Check sheet for the modelled part. Datum: model origin and axes. Units: mm. A direction names the side the tool comes from. Give positions to 0.01 mm unless a question says otherwise; leave off trailing zeros. Write each loop counter-clockwise with the first axis right and the second up, starting at its lowest first coordinate (ties: lowest second). Pieces come first, ordered by that corner, then holes. Notation, with made-up numbers: M 40,13.25 L 66,13.25 A34 ccw 66,49.25 Z; hole C -2.75,4 d3. An arc over 180 degrees is marked long. Use CSV: the item, a comma, the result in double quotes. Start each with the question number.
1. Cross-section at A-A, the plane x = 12. Enter the section's corners in (y, z).
2. Access from +Z, -Z, +X, -X, +Y, -Y to the whole of each face (thin tool, end or side, straight path). Record for faces 4 (the face through (15, 13, -7.62)), 5 (the face through (9.144, 1, -33)), 6 (the face through (19.05, 1, -61)), 7 (the face through (18.84, 21.43, -33.12)), 8 (the face through (8.37, 3.06, -33.12)).
3. Mould release check, pull along X, two halves, no side actions. Record for faces 1 (the face through (31, 3, -7.62)), 2 (the face through (32.84, 1.13, -53.83)), 3 (the face through (7.62, 12, -33)): +X half, -X half, draft (parallel to the pull), parting line (faces both ways), or undercut.
4. Scan lines: line 1 (Z direction, x = 9, y = 17.75); line 2 (Y direction, x = 34.5, z = -22.5); line 3 (X direction, y = 8, z = -40). Record each from-to range of solid material in increasing order.
5. Cross-section at B-B, the plane z = -36. Enter the section's corners in (x, y), and give its area (3 significant figures).
6. Cross-section at D-D, the plane z = -23. Enter the section's corners in (x, y), and give its area (3 significant figures).
7. Cross-section at C-C, the plane x = 5. Enter the section's corners in (y, z).
8. Depth check by flat-ended pin: P1, Ø2.5, axis at x = 29.5, z = -5.5, coming from the +Y side; P2, Ø7, axis at x = 16, y = 14.5, coming from the -Z side; P3, Ø4, axis at x = 4, y = 20, coming from the +Z side; P4, Ø4, axis at y = 9, z = -22.5, coming from the +X side. Enter the tip coordinate at first touch or a pass-through.
from build123d import *

# Parameters (mm, degrees)
BOSS_EXTRUDE2_DEPTH   = 3.81
BOSS_EXTRUDE2_2_DEPTH = 3.81
SKETCH2_3_W           = 39.3827
SKETCH2_3_H           = 60.96
SKETCH2_3_R           = 2.794
SKETCH2_3_W_2         = 7.874
SKETCH2_3_H_2         = 50.8
BOSS_EXTRUDE3_DEPTH   = 2.286
SKETCH2_4_W           = 0.75
SKETCH2_4_H           = 50.8
BOSS_EXTRUDE4_DEPTH   = 22.86
SKETCH7_W             = 50.8
SKETCH7_H             = 0.889
BOSS_EXTRUDE6_DEPTH   = 12.7
BOSS_EXTRUDE7_DEPTH   = 0.889
BOSS_EXTRUDE8_DEPTH   = 50.8
SKETCH10_W            = 11.873277716
SKETCH10_H            = 49.911
CUT_EXTRUDE5_DEPTH    = 89.208426668


with BuildPart() as part:
    # Sketch2 → Boss-Extrude2 (new body)
    with BuildSketch(Plane(origin=(0, 0, 0), x_dir=(1, 0, 0), z_dir=(0, 1, 0))):
        Polygon((0, 7.62), (0, 0), (39.3827, 0), (39.3827, 7.62), (7.62, 7.62), (6.87, 7.62), align=None)
    extrude(amount=BOSS_EXTRUDE2_DEPTH)



with BuildPart() as body_2:
    # Sketch2 → Boss-Extrude2 2 (new body)
    with BuildSketch(Plane(origin=(0, 0, 0), x_dir=(1, 0, 0), z_dir=(0, 1, 0))):
        Polygon((0, 76.2), (0, 68.58), (6.87, 68.58), (7.62, 68.58), (39.3827, 68.58), (39.3827, 76.2), align=None)
    extrude(amount=BOSS_EXTRUDE2_2_DEPTH)


with BuildPart() as part_1:
    add(part.part)

    add(body_2.part)  # Boss-Extrude3 merges body 2
    # Sketch2<3> → Boss-Extrude3 (add)
    with BuildSketch(Plane(origin=(0, 0, 0), x_dir=(1, 0, 0), z_dir=(0, 1, 0))):
        with Locations((19.69135, 38.1)):
            Rectangle(SKETCH2_3_W, SKETCH2_3_H)
        with Locations(Location((30.067932262, 53.467, 0), (0, 0, 270))):
            Circle(SKETCH2_3_R, mode=Mode.SUBTRACT)
        with Locations((15.113, 38.1)):
            Rectangle(SKETCH2_3_W_2, SKETCH2_3_H_2, mode=Mode.SUBTRACT)
        with Locations(Location((30.067932262, 22.733, 0), (0, 0, 270))):
            Circle(SKETCH2_3_R, mode=Mode.SUBTRACT)
    extrude(amount=BOSS_EXTRUDE3_DEPTH)

    # Sketch2<4> → Boss-Extrude4 (add)
    with BuildSketch(Plane(origin=(0, 0, 0), x_dir=(1, 0, 0), z_dir=(0, 1, 0))):
        with Locations((7.245, 33.02)):
            Rectangle(SKETCH2_4_W, SKETCH2_4_H)
    extrude(amount=BOSS_EXTRUDE4_DEPTH)

    # Sketch7 → Boss-Extrude6 (add)
    with BuildSketch(Plane(origin=(7.62, 0, 0), x_dir=(0, 0, -1), z_dir=(1, 0, 0))):
        with Locations((33.02, 22.4155)):
            Rectangle(SKETCH7_W, SKETCH7_H)
    extrude(amount=BOSS_EXTRUDE6_DEPTH)

    # Sketch8 → Boss-Extrude7 (add)
    with BuildSketch(Plane(origin=(0, 0, -7.62), x_dir=(-1, 0, 0), z_dir=(0, 0, -1))):
        Polygon((-21.895037632, 3.81), (-7.62, 3.81), (-7.62, 20.64426719), (-8.94673281, 21.971), (-17.961616695, 21.971), (-19.689000062, 20.906791166), align=None)
        Polygon((-21.017277716, 2.286), (-21.895037632, 3.81), (-22.091682793, 2.286), align=None)
        Polygon((-9.144, 2.286), (-7.62, 2.286), (-7.62, 3.81), align=None)
        Polygon((-8.94673281, 21.971), (-7.62, 20.64426719), (-7.62, 21.971), align=None)
        Polygon((-19.551682793, 21.971), (-19.689000062, 20.906791166), (-17.961616695, 21.971), align=None)
        Polygon((-9.144, 2.286), (-7.62, 3.81), (-21.895037632, 3.81), (-21.017277716, 2.286), align=None)
    extrude(amount=BOSS_EXTRUDE7_DEPTH)

    # Sketch8<4> → Boss-Extrude8 (add)
    with BuildSketch(Plane(origin=(0, 0, -7.62), x_dir=(-1, 0, 0), z_dir=(0, 0, -1))):
        Polygon((-22.663354839, 3.81), (-21.895037632, 3.81), (-19.689000062, 20.906791166), (-19.551682793, 21.971), (-20.32, 21.971), align=None)
        Polygon((-22.091682793, 2.286), (-21.895037632, 3.81), (-22.663354839, 3.81), (-22.86, 2.286), align=None)
        Polygon((-21.017277716, 2.286), (-21.895037632, 3.81), (-22.091682793, 2.286), align=None)
        Polygon((-9.144, 2.286), (-7.62, 2.286), (-7.62, 3.81), align=None)
        Polygon((-19.551682793, 21.971), (-19.689000062, 20.906791166), (-17.961616695, 21.971), align=None)
        Polygon((-8.94673281, 21.971), (-7.62, 20.64426719), (-7.62, 21.971), align=None)
    extrude(amount=BOSS_EXTRUDE8_DEPTH)

    # Sketch10 → Cut-Extrude5 (cut, through all)
    with BuildSketch(Plane(origin=(0, 2.286, 0), x_dir=(1, 0, 0), z_dir=(0, 1, 0))):
        with Locations((15.080638858, 33.4645)):
            Rectangle(SKETCH10_W, SKETCH10_H)
    extrude(amount=-CUT_EXTRUDE5_DEPTH, mode=Mode.SUBTRACT)


solid = part_1.part
Worked answers:
1,outline,"M 0,-76.2 L 3.81,-76.2 L 3.81,-68.58 L 2.29,-68.58 L 2.29,-63.5 L 0,-63.5 Z; M 0,-8.51 L 21.97,-8.51 L 21.97,-58.42 L 22.86,-58.42 L 22.86,-7.62 L 3.81,-7.62 L 3.81,0 L 0,0 Z"
2,face 4,"+Z, +X, -X, +Y"
2,face 5,"-Y"
2,face 6,"+Y, -Y"
2,face 7,"-Z, -Y"
2,face 8,"none"
3,face 1,"draft"
3,face 2,"undercut"
3,face 3,"undercut"
4,line 1,"z = -8.51 to -7.62"
4,line 2,"y = 0 to 2.29"
4,line 3,"x = 6.87 to 7.62, 21.35 to 22.12"
5,outline,"M 0,0 L 9.14,0 L 9.14,2.29 L 7.62,3.81 L 7.62,20.64 L 8.95,21.97 L 17.96,21.97 L 19.69,20.91 L 21.9,3.81 L 21.02,2.29 L 21.02,0 L 39.38,0 L 39.38,2.29 L 22.86,2.29 L 20.32,21.97 L 20.32,22.86 L 6.87,22.86 L 6.87,2.29 L 0,2.29 Z"
5,area,"108 mm^2"
6,outline,"M 0,0 L 9.14,0 L 9.14,2.29 L 7.62,3.81 L 7.62,20.64 L 8.95,21.97 L 17.96,21.97 L 19.69,20.91 L 21.9,3.81 L 21.02,2.29 L 21.02,0 L 27.29,0 L 27.29,2.29 L 22.86,2.29 L 20.32,21.97 L 20.32,22.86 L 6.87,22.86 L 6.87,2.29 L 0,2.29 Z; M 32.85,0 L 39.38,0 L 39.38,2.29 L 32.85,2.29 Z"
6,area,"95.7 mm^2"
7,outline,"M 0,-76.2 L 3.81,-76.2 L 3.81,-68.58 L 2.29,-68.58 L 2.29,-7.62 L 3.81,-7.62 L 3.81,0 L 0,0 Z"
8,P1,"stops at y = 3.81"
8,P2,"stops at z = -8.51"
8,P3,"passes through"
8,P4,"stops at x = 22.25"
